Could you check a few things on this model? Use its own coordinates, in mm. Face numbers are marked on the shaded views. Give positions to 0.01 mm unless a question says otherwise; leave off trailing zeros. Loops run counter-clockwise (first coordinate to the right, second up) from the corner with the lowest first, then second, coordinate; pieces in that order, holes last.
1. Thinking about a two-plate mould opening in Y: for the marked faces 1, 2 and 3, which applies, +Y half, -Y half, draft (parallel to the pull), parting line (faces both ways), or undercut?
2. For P1, Ø3, axis at y = 29, z = -1.5, coming from the -X side; P2, Ø8, axis at x = -13.5, y = 37, coming from the -Z side; P3, Ø10, axis at x = -13.5, z = 8, coming from the +Y side, each with a flat end and sliding along its axis, tell me the tip position at first contact or that it passes through.
3. Imagine slicing it at C-C (x = -9). List the corners of the cut face in (y, z) for me.
4. Imagine slicing it at B-B (y = 0). List the corners of the cut face in (x, z) for me.
5. Imagine slicing it at A-A (z = 0). List the corners of the cut face in (x, y) for me.
6. I need wall thicknesses on line 1 along Y through (x, z) = (-1.15, 0); line 2 along Z through (x, y) = (-37, 0.5). Which ranges of each line are inside material? Lowest first, please.
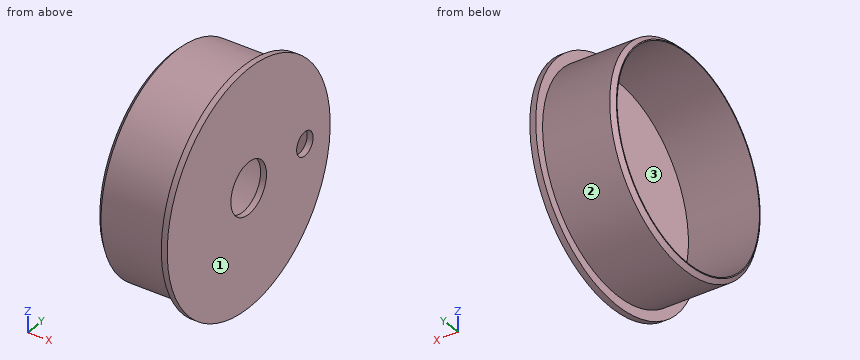
Autodesk Inventor part; units mm, degrees
ref_plane "YZ Plane" through (0, 0, 0) normal (1, 0, 0) x (0, 1, 0)
ref_plane "XZ Plane" through (0, 0, 0) normal (0, 1, 0) x (-1, 0, 0)
ref_plane "XY Plane" through (0, 0, 0) normal (0, 0, 1) x (1, 0, 0)
sketch "Sketch1" plane through (0, 0, 0) normal (0, 1, 0) x (-1, 0, 0)
  line L0 (0, 0) -> (0, -59.5)
  line L1 (0, -59.5) -> (3, -59.5)
  line L2 (3, -59.5) -> (3, -54.5)
  line L3 (3, -54.5) -> (39, -54.5)
  line L4 (39, -54.5) -> (39, -52)
  line L5 (39, -52) -> (3, -52)
  line L6 (3, -52) -> (3, 0)
  line L7 (3, 0) -> (0, 0)
  dimension "d3" = 3
  dimension "d4" = 5
  dimension "d5" = 36
  dimension "d6" = 2.5
  dimension "d14" = 52
revolve "Revolution1" add sketch "Sketch1" angle 360 about axis through (-3, 0, 0) along (1, 0, 0)
chamfer "Chamfer1" distance 2 angle 45 1 edges at (-39, 0, 54.5)
sketch "Sketch3" plane through (0, 0, 0) normal (1, 0, 0) x (0, 0, -1)
  circle A0 centre (0, 0) radius 13
  circle A1 centre (0, 0) radius 52 construction
  line L0 (0, 0) -> (0, 103.7887) construction
  circle A2 centre (0, 41) radius 6
  point P0 (0, 52)
  dimension "d15" = 26
  dimension "d16" = 12
  dimension "d17" = 11
extrude "holes" cut sketch "Sketch3" against normal blind 10
properties part number "aftPlug" material "PVC-Piping"
Derived:
1. face 1: draft
1. face 2: parting line
1. face 3: undercut
2. P1: stops at x = -3
2. P2: stops at z = -43.37
2. P3: stops at y = 54.42
3. outline: circle Ø109 at (0, 0); hole circle Ø104 at (0, 0)
4. outline: (-39, -52.5) - (-37, -54.5) - (-3, -54.5) - (-3, -59.5) - (0, -59.5) - (0, -13) - (-3, -13) - (-3, -52) - (-39, -52) - close; (-39, 52) - (-3, 52) - (-3, 13) - (0, 13) - (0, 59.5) - (-3, 59.5) - (-3, 54.5) - (-37, 54.5) - (-39, 52.5) - close
5. outline: (-39, -52.5) - (-37, -54.5) - (-3, -54.5) - (-3, -59.5) - (0, -59.5) - (0, -13) - (-3, -13) - (-3, -52) - (-39, -52) - close; (-39, 52) - (-3, 52) - (-3, 47) - (0, 47) - (0, 59.5) - (-3, 59.5) - (-3, 54.5) - (-37, 54.5) - (-39, 52.5) - close; (-3, 13) - (0, 13) - (0, 35) - (-3, 35) - close
6. line 1: y = -59.5 to -13, 13 to 35, 47 to 59.5
6. line 2: z = -54.5 to -52, 52 to 54.5
